```python
from build123d import *

# Parameters (mm, degrees)
F1_DEPTH = 1.5


with BuildPart() as f1:
    # F0 (on Top) → F1 (new body)
    with BuildSketch(Plane.XY):
        with BuildLine():
            Line((-78.070531, -28.981596), (83.511818, -28.981596))
            ThreePointArc((83.511818, -28.981596), (97.015282, 20.627403), (82.488377, 69.94642))
            Line((82.488377, 69.94642), (-77.047091, 69.94642))
            ThreePointArc((-77.047091, 69.94642), (-91.573996, 20.627403), (-78.070531, -28.981596))
        make_face()
        with BuildLine():
            ThreePointArc((-69.221243, 15.378748), (-56.875674, 41.011571), (-29.456094, 48.602439))
            ThreePointArc((-29.456094, 48.602439), (-28.318317, 45.950127), (-30.804796, 44.484958))
            ThreePointArc((-30.804796, 44.484958), (-30.30087, 43.439414), (-29.456094, 42.643514))
            ThreePointArc((-29.456094, 42.643514), (-29.754967, 38.52182), (-31.307008, 34.691826))
            ThreePointArc((-31.307008, 34.691826), (-33.073301, 34.263475), (-33.198223, 32.450281))
            ThreePointArc((-33.198223, 32.450281), (-37.743701, 31.443683), (-42.059347, 29.697312))
            ThreePointArc((-42.059347, 29.697312), (-50.547741, 20.474948), (-54.49114, 8.577283))
            ThreePointArc((-54.49114, 8.577283), (-53.878072, 3.53006), (-50.218977, 0))
            ThreePointArc((-50.218977, 0), (-44.019674, 2.905988), (-41.092087, 9.09512))
            ThreePointArc((-41.092087, 9.09512), (-41.596159, 9.931856), (-42.516142, 10.260256))
            Line((-42.516142, 10.260256), (-45.299519, 10.260256))
            ThreePointArc((-45.299519, 10.260256), (-47.249951, 14.121331), (-44.263843, 17.251067))
            ThreePointArc((-44.263843, 17.251067), (-43.416051, 17.995459), (-44.263843, 18.739851))
            ThreePointArc((-44.263843, 18.739851), (-44.75679, 21.306075), (-42.580869, 22.753095))
            Line((-42.580869, 22.753095), (-26.139516, 22.753095))
            ThreePointArc((-26.139516, 22.753095), (-23.806404, 22.144728), (-23.097219, 19.840257))
            Line((-23.097219, 19.840257), (-24.780193, 11.945932))
            ThreePointArc((-24.780193, 11.945932), (-25.908191, 10.415742), (-27.723249, 9.850567))
            ThreePointArc((-27.723249, 9.850567), (-29.192747, 4.809992), (-31.297695, 0))
            ThreePointArc((-31.297695, 0), (-40.716383, -9.995095), (-54.100201, -13.075197))
            ThreePointArc((-54.100201, -13.075197), (-66.483065, -3.568669), (-68.217009, 11.945932))
            ThreePointArc((-68.217009, 11.945932), (-68.068902, 13.852556), (-69.221243, 15.378748))
        make_face(mode=Mode.SUBTRACT)
        with BuildLine():
            ThreePointArc((-21.219255, -12.345982), (-19.944396, 10.29328), (-15.124779, 32.450281))
            ThreePointArc((-15.124779, 32.450281), (-16.238245, 32.156524), (-17.377038, 32.327555))
            ThreePointArc((-17.377038, 32.327555), (-17.701466, 37.582362), (-15.762346, 42.47706))
            ThreePointArc((-15.762346, 42.47706), (-15.39411, 45.513529), (-13.340303, 47.78016))
            Line((-13.340303, 47.78016), (17.581943, 47.78016))
            ThreePointArc((17.581943, 47.78016), (19.376598, 47.456686), (20.675082, 46.176311))
            Line((20.675082, 46.176311), (19.60909, 38.391046))
            ThreePointArc((19.60909, 38.391046), (18.718733, 37.856487), (17.703688, 37.637003))
            ThreePointArc((17.703688, 37.637003), (19.077047, 34.545895), (16.411087, 32.464135))
            Line((16.411087, 32.464135), (2.676149, 32.464135))
            ThreePointArc((2.676149, 32.464135), (0.993774, 27.613666), (0, 22.576816))
            Line((0, 22.576816), (9.333577, 22.576816))
            ThreePointArc((9.333577, 22.576816), (11.379026, 16.571914), (8.8095, 10.771892))
            ThreePointArc((8.8095, 10.771892), (7.828648, 9.973453), (6.596562, 9.687897))
            Line((6.596562, 9.687897), (-3.560899, 9.687897))
            ThreePointArc((-3.560899, 9.687897), (-6.91927, -1.159813), (-8.874034, -12.345982))
            ThreePointArc((-8.874034, -12.345982), (-15.046644, -13.81701), (-21.219255, -12.345982))
        make_face(mode=Mode.SUBTRACT)
        with BuildLine():
            ThreePointArc((24.318619, -13.598498), (22.572563, -12.506763), (22.547672, -10.447643))
            Line((22.547672, -10.447643), (37.622835, 17.960656))
            Line((37.622835, 17.960656), (28.403541, 44.209484))
            ThreePointArc((28.403541, 44.209484), (28.605897, 46.528204), (30.480955, 47.907177))
            ThreePointArc((30.480955, 47.907177), (37.950305, 48.319326), (45.419656, 47.907177))
            ThreePointArc((45.419656, 47.907177), (46.387462, 46.960221), (46.68678, 45.639697))
            Line((46.68678, 45.639697), (48.554119, 35.102576))
            Line((48.554119, 35.102576), (55.289872, 44.839408))
            ThreePointArc((55.289872, 44.839408), (57.776817, 47.408886), (60.958575, 49.040917))
            Line((60.958575, 49.040917), (72.734997, 48.503447))
            ThreePointArc((72.734997, 48.503447), (74.349534, 47.270892), (73.76077, 45.326855))
            Line((73.76077, 45.326855), (35.466932, -13.432029))
            ThreePointArc((35.466932, -13.432029), (29.89986, -13.989714), (24.318619, -13.598498))
        make_face(mode=Mode.SUBTRACT)
    extrude(amount=F1_DEPTH)


solid = f1.part
```
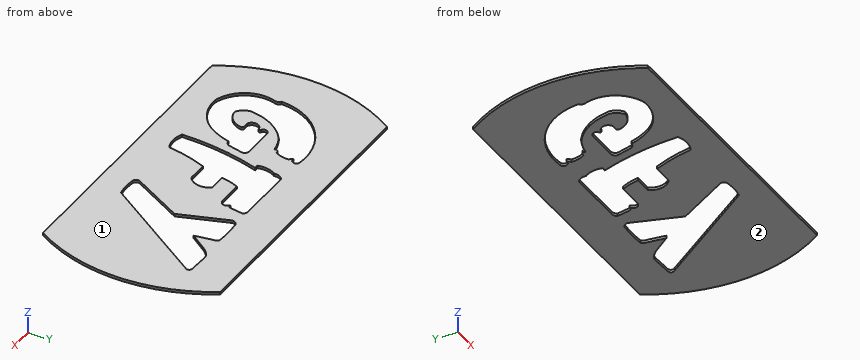
Source: CAD feature listing. Evaluate the final solid. Frame: model axes, mm. Face numbers are marked on the shaded views. Coordinates: 2 decimals unless noted, no trailing zeros. Order: outer loops, then holes, each group sorted by start corner. A loop starts at its lowest first (then second) coordinate and runs counter-clockwise, first axis right, second up. Notation, with made-up numbers: (-6, -20.5) - (-2, -20.5) arc R24 cw to (-2, 11.5) - close; hole circle Ø6 at (61, 2). An arc over 180 degrees is marked (long way). One line per item, written item: value.
1) Cut plane B-B on x = -38.5. Output: boundary loops of the cut face in (y, z).
Computed values:
outline: (-28.98, 0) - (-8.55, 0) - (-8.55, 1.5) - (-28.98, 1.5) - close; (22.75, 0) - (31.2, 0) - (31.2, 1.5) - (22.75, 1.5) - close; (48.82, 0) - (69.95, 0) - (69.95, 1.5) - (48.82, 1.5) - close
2) Cut plane A-A on y = -5. Output: boundary loops of the cut face in (x, z).
Computed values:
outline: (-88.3, 0) - (-65.59, 0) - (-65.59, 1.5) - (-88.3, 1.5) - close; (-34.64, 0) - (-21.2, 0) - (-21.2, 1.5) - (-34.64, 1.5) - close; (-7.76, 0) - (25.44, 0) - (25.44, 1.5) - (-7.76, 1.5) - close; (40.96, 0) - (93.74, 0) - (93.74, 1.5) - (40.96, 1.5) - close
3) Cut plane C-C on z = 1.2. State how many separate pieces and enclosed holes the cut face has, plus the area to 3 significant figures.
Computed values:
separate pieces: 1
enclosed holes: 3
area: 13,100 mm^2
4) Mould query, pull axis Z, two halves, no side actions, for the marked faces 1 and 2. Classes: released by +Z, released by -Z, zero draft, split by the parting line, or undercut.
Computed values:
face 1: released by +Z
face 2: released by -Z
5) Ray query, line 1 (Y direction, x = 4, z = 0.15); line 2 (X direction, y = 13, z = 1.3); line 3 (Y direction, x = -47, z = 1.1). Return the intervals inside material, ascending. Write a range as [from, to].
Computed values:
line 1: y = [-28.98, 9.69], [22.58, 32.46], [47.78, 69.95]
line 2: x = [-91.34, -67.96], [-53.67, -47.25], [-24.56, -19.55], [10.44, 34.99], [52.69, 96.79]
line 3: y = [-28.98, -12.49], [0.85, 12.12], [15.02, 25.31], [46.79, 69.95]
